Solid Edge part; units mm, degrees
sketch "Sketch1" plane through (0, 0, 0) normal (0, -1, 0) x (1, 0, 0)
  circle A0 centre (0, 0) radius 12.5
extrude "Protrusion1" add sketch "Sketch1" against normal blind 30
sketch "Sketch2" plane through (0, 30, 0) normal (0, 1, 0) x (-1, 0, 0)
  circle A0 centre (0, 0) radius 7.5
extrude "ExtrudedProtrusion_2" add sketch "Sketch2" along normal blind 30
sketch "Sketch3" plane through (0, 60, 0) normal (0, 1, 0) x (-1, 0, 0)
  circle A0 centre (0, 0) radius 7.5
extrude "ExtrudedProtrusion_3" add sketch "Sketch3" along normal blind 510
Work out the finished part from the listing and answer in its coordinate system (mm). A direction names the side the tool comes from. Give positions to 0.01 mm unless a question says otherwise; leave off trailing zeros. Order: outer loops, then holes, each group sorted by start corner. A loop starts at its lowest first (then second) coordinate and runs counter-clockwise, first axis right, second up. Notation, with made-up numbers: (-31, -26) -> (15, -26) arc R9 ccw to (15, -15) -> close; hole circle Ø8 at (-11.5, 58). An arc over 180 degrees is marked (long way). One line per item, written item: value.
Item 1: Straight lines are drawn through the part: probe 1 along X at (y, z) = (210.5, 0.5); probe 2 along Y at (x, z) = (-1.5, -7.5). For each, find the intervals that lie inside material, in ascending order.
Answer sheet:
probe 1: -7.48 to 7.48
probe 2: 0 to 30
Item 2: Find section B-B, the plane z = 0. Give the vertices of the cut face in (x, y).
Answer sheet:
outline: (-12.5, 0) -> (12.5, 0) -> (12.5, 30) -> (7.5, 30) -> (7.5, 570) -> (-7.5, 570) -> (-7.5, 30) -> (-12.5, 30) -> close
Item 3: Flat-ended cylindrical pins translate along their axes: P1, Ø5, axis at x = -10, z = 7.5, coming from the +Y side; P2, Ø1.5, axis at y = 291.5, z = -2, coming from the +X side; P3, Ø8, axis at y = 322.5, z = 0, coming from the +X side. Find the tip coordinate at first contact, or state that the pin passes through.
Answer sheet:
P1: y = 30
P2: x = 7.4
P3: x = 7.5
Item 4: Find section A-A, the plane x = 0. Give the vertices of the cut face in (y, z).
Answer sheet:
outline: (0, -12.5) -> (30, -12.5) -> (30, -7.5) -> (570, -7.5) -> (570, 7.5) -> (30, 7.5) -> (30, 12.5) -> (0, 12.5) -> close
Item 5: A tool of negligible diameter and unlimited length cuts with its end or side. For faces 1 (the flat face through (-8, 30, 0)), 2 (the flat face through (0, 570, 0)), from which of +Z, -Z, +X, -X, +Y, -Y can it reach the whole face along a straight path? Write none if from no direction.
Answer sheet:
face 1: +Y
face 2: +Z, -Z, +X, -X, +Y
Item 6: Find section C-C, the plane y = 213.5. Give the vertices of the cut face in (x, z), plus the area to 3 significant figures.
Answer sheet:
outline: circle Ø15 at (0, 0)
area: 177 mm²
